Source: three-view drawing plus pictorial views. Frame: mm from the lowest corner of the part. A direction names the side the tool comes from. Give positions to 0.01 mm unless a question says otherwise; leave off trailing zeros. Order: outer loops, then holes, each group sorted by start corner. A loop starts at its lowest first (then second) coordinate and runs counter-clockwise, first axis right, second up. Notation, with made-up numbers: (49.5, -20) - (96.5, -20) arc R19 cw to (96.5, -4) - close; hole circle Ø6 at (70.25, -4.5). An arc over 180 degrees is marked (long way). Answer in a Markdown table with one row per item. Add a question column.
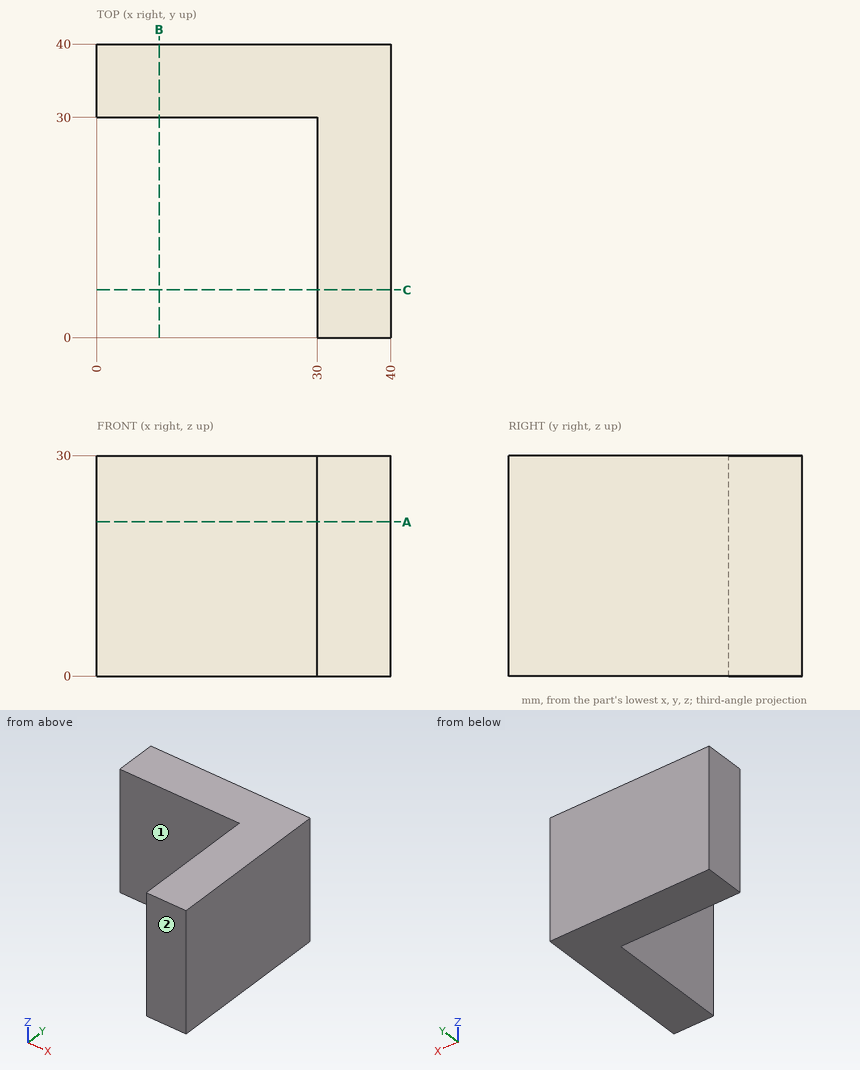
Q1. Access query for the marked faces 1 and 2. Directions: +Z, -Z, +X, -X, +Y, -Y. A direction counts if a zero-diameter tool reaches every point of the face in a straight line with its end or side. Return the directions, or none.
Q2. Section B-B, the plane x = 8.5. Return loops of the section in (y, z).
Q3. Contact query for flat-ended pins moving along their axis: P1, Ø5, axis at x = 10.5, z = 7.5, coming from the -Y side; P2, Ø5, axis at x = 5.5, y = 29, coming from the +Z side; P3, Ø2, axis at y = 5.5, z = 22.5, coming from the -X side. Output: stop coordinate, or through.
Q4. Section A-A, the plane z = 21. Return loops of the section in (x, y), then the cut area to 3 significant figures.
Q5. Line query: probe 1 along Y at (x, z) = (4.5, 25.25). Output: solid intervals per line, ascending.
Computed:
| question | item | result |
|---|---|---|
| 1 | face 1 | +Z, -Z, -X, -Y |
| 1 | face 2 | +Z, -Z, +X, -X, -Y |
| 2 | outline | (30, 0) - (40, 0) - (40, 30) - (30, 30) - close |
| 3 | P1 | stops at y = 30 |
| 3 | P2 | stops at z = 30 |
| 3 | P3 | stops at x = 30 |
| 4 | outline | (0, 30) - (30, 30) - (30, 0) - (40, 0) - (40, 40) - (0, 40) - close |
| 4 | area | 700 mm^2 |
| 5 | probe 1 | y = 30 to 40 |
